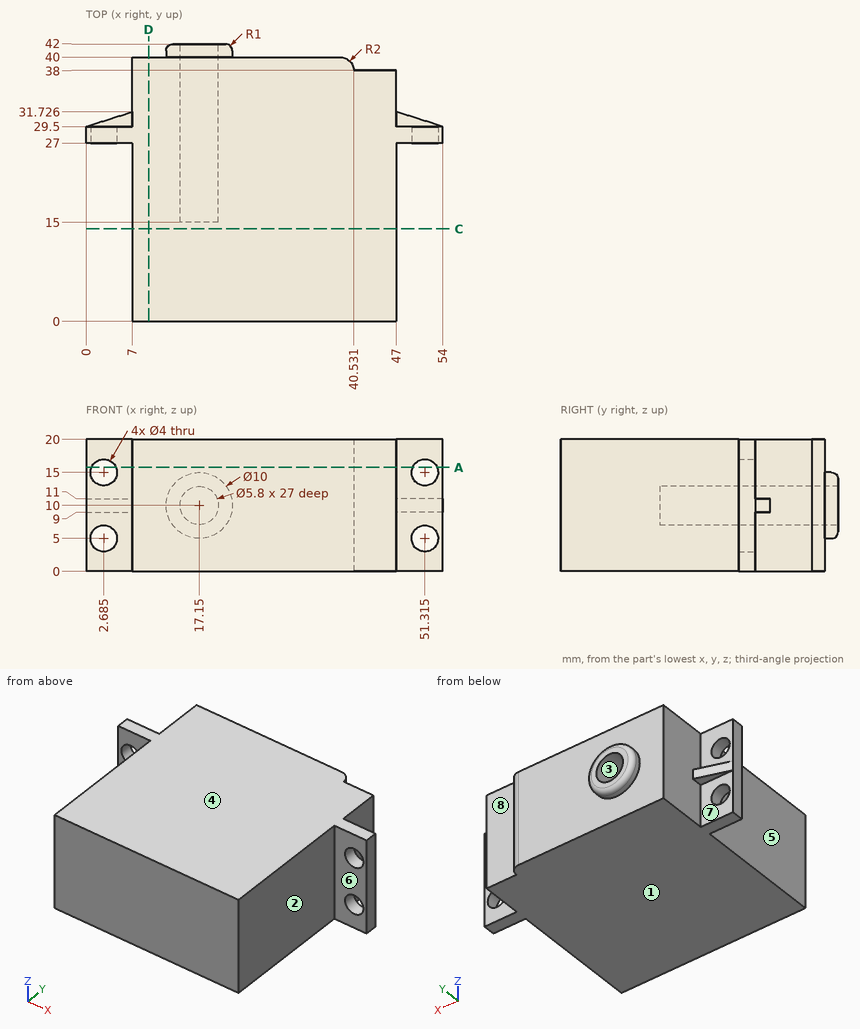
Geometry check sheet. Reference: drawing and pictorial views, mm from the part's lowest x, y, z. A direction names the side the tool comes from. Give positions to 0.01 mm unless a question says otherwise; leave off trailing zeros. Order: outer loops, then holes, each group sorted by start corner. A loop starts at its lowest first (then second) coordinate and runs counter-clockwise, first axis right, second up. Notation, with made-up numbers: (85.5, 30) -> (128.5, 30) arc R27 cw to (128.5, 65) -> close; hole circle Ø1 at (77, -7). An arc over 180 degrees is marked (long way). Write each question's results on one line, items separated by ' | '. Start each with the question number.
(1) Gauge pin test, flat ends, axial feed: P1, Ø12, axis at y = 9, z = 13.5, coming from the -X side; P2, Ø7.5, axis at x = 3, z = 16, coming from the +Y side; P3, Ø12, axis at x = 28.5, z = 4, coming from the +Y side; P4, Ø3, axis at x = 2.685, z = 5, coming from the +Y side. Record the tip position at first contact, or that the pin passes through.
(2) Access from +Z, -Z, +X, -X, +Y, -Y to the whole of each face (thin tool, end or side, straight path). Record for the marked faces 4, 5, 6, 7 and 8.
(3) Sectioned sample at C-C (y = 14). Enter the section's corners in (x, z), plus the area to 3 significant figures.
(4) Scan lines: line 1 (X direction, y = 28.9, z = 5) (1 decimal); line 2 (Y direction, x = 5, z = 8.25); line 3 (X direction, y = 13, z = 6.75). Record each from-to range of solid material in increasing order.
(5) Mould release check, pull along X, two halves, no side actions. Record for the marked faces 1, 2 and 3: pulls with the +X half, pulls with the -X half, needs draft (parallel to the pull), parting line crosses it, or undercut.
(6) Sectioned sample at A-A (z = 15.75). Give the number of separate pieces and of enclosed holes in the cut face, plus the area to 3 significant figures.
(7) Sectioned sample at D-D (x = 9.5). Enter the section's corners in (y, z).
Answer below:
1) P1: x = 7 | P2: y = 29.5 | P3: y = 40 | P4: through
2) face 4: +Z, +X, -X, +Y, -Y | face 5: +Z, -Z, -X, -Y | face 6: +Z, -Z, +X, -Y | face 7: -Z, -X, +Y | face 8: +Z, -Z, +X, +Y
3) outline: (7, 0) -> (47, 0) -> (47, 20) -> (7, 20) -> close | area: 800 mm2
4) line 1: 0 to 0.7, 4.7 to 49.3, 53.3 to 54 | line 2: 27 to 29.5 | line 3: 7 to 47
5) face 1: needs draft | face 2: pulls with the +X half | face 3: undercut
6) separate pieces: 3 | enclosed holes: 0 | area: 1,600 mm2
7) outline: (0, 0) -> (40, 0) -> (40, 20) -> (0, 20) -> close
